from build123d import *

# Parameters (mm, degrees)
F0_R     = 5.0165
F0_R_2   = 4.0005
F1_DEPTH = 76.2
F3_DEPTH = 8.4836
F5_DEPTH = 25.4
F7_DEPTH = 3.175
F8_W     = 8.4836
F8_H     = 3.175
F9_DEPTH = 6.35


# Not quite as in the source:
# - ends of sketch curves that miss each other by under 0.0002 mm in the source are joined


with BuildPart() as f1:
    # F0 (on Top) → F1 (new body)
    with BuildSketch(Plane.XY):
        Circle(F0_R)
        Circle(F0_R_2, mode=Mode.SUBTRACT)
    extrude(amount=F1_DEPTH)

    # F2 (on face) → F3 (join)
    with BuildSketch(Plane.XY.offset(76.2)):
        Polygon((-4.2418, -22.9430834), (0, -22.9430834), (4.2418, -22.9430834), (4.2418, -19.7680834), (1.5875, -19.7680834), (1.5875, -5.0165), (1.5875, -4.7586884748), (0, -4.7586884748), (-1.5875, -4.7586884748), (-1.5875, -19.7680834), (-4.2418, -19.7680834), align=None)
    extrude(amount=-F3_DEPTH)

    # F4 (on face) → F5 (cut)
    with BuildSketch(Plane.YZ.offset(1.5875)):
        with BuildLine():
            Line((-4.7586884748, 69.4789886475), (-4.7586884748, 74.6846720576))
            ThreePointArc((-4.7586884748, 74.6846720576), (-6.34993848, 72.0818303525), (-4.7586884748, 69.4789886475))
        make_face()
    extrude(amount=-F5_DEPTH, mode=Mode.SUBTRACT)

    # F6 (on face) → F7 (join)
    with BuildSketch(Plane.XY.offset(76.2)):
        Polygon((4.2418, -21.3555831969), (4.2418, -22.9430834), (18.1297326, -22.9430831969), (21.3047326, -22.9430831969), (21.3047326, -22.2236789969), (21.3047326, -15.8736789969), (14.9547326, -15.8736789969), (14.9547326, -21.3555831969), align=None)
        with BuildLine():
            ThreePointArc((18.1297326, -20.3186789969), (17.2317069879, -18.1506533848), (19.3997326, -19.0486789969))
            ThreePointArc((19.3997326, -19.0486789969), (19.0277582121, -19.946704609), (18.1297326, -20.3186789969))
        make_face(mode=Mode.SUBTRACT)
        Polygon((-4.2418, -22.9430831969), (0, -22.9430831969), (4.2418, -22.9430831969), (4.2418, -21.3555831969), (-4.2418, -21.3555831969), align=None)
        Polygon((-18.1297326, -22.9430831969), (-4.2418, -22.9430831969), (-4.2418, -21.3555831969), (-14.9547326, -21.3555831969), (-14.9547326, -15.8736789969), (-21.3047326, -15.8736789969), (-21.3047326, -22.2236789969), (-21.3047326, -22.9430831969), align=None)
        with BuildLine():
            ThreePointArc((-18.1297326, -20.3186789969), (-19.0277582121, -18.1506533848), (-16.8597326, -19.0486789969))
            ThreePointArc((-16.8597326, -19.0486789969), (-17.2317069879, -19.946704609), (-18.1297326, -20.3186789969))
        make_face(mode=Mode.SUBTRACT)
    extrude(amount=-F7_DEPTH)

    # F8 (on face) → F9 (join)
    with BuildSketch(Plane(origin=(0, 0, 67.7164), x_dir=(1, 0, 0), z_dir=(0, 0, -1))):
        with Locations((0, 21.3555834)):
            Rectangle(F8_W, F8_H)
    extrude(amount=F9_DEPTH)


solid = f1.part
The model under review builds one solid part; all positions refer to its coordinate system, in mm. A direction names the side the tool comes from. Coordinates: 2 decimals unless noted, no trailing zeros. Write each loop counter-clockwise with the first axis right and the second up, starting at its lowest first coordinate (ties: lowest second). Pieces come first, ordered by that corner, then holes. Notation, with made-up numbers: (35, 77) - (88, 77) arc R30 cw to (88, 99) - close; hole circle Ø4 at (-18.5, 33). An arc over 180 degrees is marked (long way). Answer as a JSON object with one key per item and string values. Group by question number.
1. Add section A-A (x = 0). Give the boundary of the cut face in (y, z).
2. Clearance check with flat-ended pins moving along their axes: pin 1 Ø1.6 at (x, y) = (-0.5, -12.5) entering from -Z; pin 2 Ø3.5 at (x, y) = (2, -21.5) entering from -Z; pin 3 Ø4 at (y, z) = (-11.5, 72) entering from -X. State where each tip first meets the part, or that it passes through.
3. Add section B-B (y = 0). Give the boundary of the cut face in (x, z).
4. Add section D-D (z = 26). Give the boundary of the cut face in (x, y).
5. Machinability: for faces 1 (the face through (-14.955, -19, 75)), 2 (the face through (18, -15.874, 75)), 3 (the face through (0, -19.768, 67)), 4 (the face through (-18, -15.874, 75)), 5 (the face through (0, -21, 61.366)), which of the approach directions +Z, -Z, +X, -X, +Y, -Y give a long, thin tool a straight path to every point of the face, cutting with its end or side? Answer none if there is none.
6. To check wall thickness, follow probe 1 along Y at (x, z) = (0, 20); probe 2 along Z at (x, y) = (-1, -9); probe 3 along Y at (x, z) = (-1, 48). State the ranges of each line that lie inside material, in increasing order.
7. Add section C-C (z = 72). Give the boundary of the cut face in (x, y), plus the area to 3 significant figures.
8. Mouldability with a two-part tool opening along Z and no side actions: class faces 6 (the face through (0, -4.759, 72)), 7 (the face through (16, -20, 73.025)), 8 (the face through (14.955, -19, 75)), 9 (the face through (0.02, -6.35, 72.13)) as pulls with the +Z half, pulls with the -Z half, needs draft (parallel to the pull), parting line crosses it, or undercut.
Findings:
{
 "1": {"outline": "(-22.94, 61.37) - (-19.77, 61.37) - (-19.77, 67.72) - (-5.02, 67.72) - (-5.02, 0) - (-4, 0) - (-4, 76.2) - (-22.94, 76.2) - close; (4, 0) - (5.02, 0) - (5.02, 76.2) - (4, 76.2) - close; hole (-4.76, 69.48) - (-4.76, 74.68) arc R2.92 ccw to start"},
 "2": {"pin 1": "z = 67.72", "pin 2": "z = 61.37", "pin 3": "x = -1.59"},
 "3": {"outline": "(-5.02, 0) - (-4, 0) - (-4, 76.2) - (-5.02, 76.2) - close; (4, 0) - (5.02, 0) - (5.02, 76.2) - (4, 76.2) - close"},
 "4": {"outline": "circle Ø10.03 at (0, 0); hole circle Ø8 at (0, 0)"},
 "5": {"face 1": "+Z, -Z, +Y", "face 2": "+Z, -Z, +X, +Y", "face 3": "-Z", "face 4": "+Z, -Z, -X, +Y", "face 5": "-Z, +X, -X, -Y"},
 "6": {"probe 1": "-5.02 to -4, 4 to 5.02", "probe 2": "67.72 to 76.2", "probe 3": "-4.92 to -3.87, 3.87 to 4.92"},
 "7": {"outline": "(-4.24, -22.94) - (4.24, -22.94) - (4.24, -19.77) - (1.59, -19.77) - (1.59, -6.35) - (-1.59, -6.35) - (-1.59, -19.77) - (-4.24, -19.77) - close; (-1.59, -4.76) - (1.59, -4.76) arc R5.02 ccw (long way) to start; hole circle Ø8 at (0, 0)", "area": "97.8 mm²"},
 "8": {"face 6": "undercut", "face 7": "pulls with the -Z half", "face 8": "needs draft", "face 9": "undercut"}
}
